from build123d import *

# Parameters (mm, degrees)
SKETCH1_W               = 406.4
SKETCH1_H               = 406.4
BOSS_EXTRUDE1_DEPTH     = 6.35
SKETCH2_R               = 50.8
CUT_EXTRUDE1_DEPTH      = 6.35
SKETCH3_W               = 406.4
SKETCH3_H               = 254
BOSS_EXTRUDE4_DEPTH     = 12.7
SKETCH6_R               = 50.8
CUT_EXTRUDE3_DEPTH      = 288.998927949
SKETCH7_R               = 7.14375
CUT_EXTRUDE4_DEPTH      = 288.648691984
F_1_2_20_TAPPED_HOLE1_D = 11.50874
SKETCH11_R              = 7.14375
CUT_EXTRUDE5_DEPTH      = 288.998927949


with BuildPart() as part:
    # Sketch1 → Boss-Extrude1 (new body)
    with BuildSketch(Plane(origin=(0, 0, 0), x_dir=(1, 0, 0), z_dir=(0, 1, 0))):
        Rectangle(SKETCH1_W, SKETCH1_H)
    extrude(amount=BOSS_EXTRUDE1_DEPTH)

    # Sketch2 → Cut-Extrude1 (cut)
    with BuildSketch(Plane(origin=(0, 6.35, 0), x_dir=(1, 0, 0), z_dir=(0, 1, 0))):
        with Locations(Location((-50.8, -55.88, 0), (0, 0, 270))):
            Circle(SKETCH2_R)
    extrude(amount=-CUT_EXTRUDE1_DEPTH, mode=Mode.SUBTRACT)

    # Sketch3 → Boss-Extrude4 (add)
    with BuildSketch(Plane(origin=(0, 6.35, 0), x_dir=(1, 0, 0), z_dir=(0, 1, 0))):
        with Locations((0, 76.2)):
            Rectangle(SKETCH3_W, SKETCH3_H)
    extrude(amount=BOSS_EXTRUDE4_DEPTH)

    # Sketch6 → Cut-Extrude3 (cut, through all)
    with BuildSketch(Plane.XZ):
        with Locations(Location((-50.8, 55.88, 0), (0, 0, 90))):
            Circle(SKETCH6_R)
    extrude(amount=-CUT_EXTRUDE3_DEPTH, mode=Mode.SUBTRACT)

    # Sketch7 → Cut-Extrude4 (cut, through all)
    with BuildSketch(Plane(origin=(0, 6.35, 0), x_dir=(1, 0, 0), z_dir=(0, 1, 0))):
        with Locations(Location((174.625, -182.5625, 0), (0, 0, 270))):
            Circle(SKETCH7_R)
        with Locations(Location((127, -182.5625, 0), (0, 0, 270))):
            Circle(SKETCH7_R)
        with Locations(Location((-174.625, -182.5625, 0), (0, 0, 270))):
            Circle(SKETCH7_R)
        with Locations(Location((-127, -182.5625, 0), (0, 0, 270))):
            Circle(SKETCH7_R)
    extrude(amount=-CUT_EXTRUDE4_DEPTH, mode=Mode.SUBTRACT)

    # 1/2-20 Tapped Hole1 (through all)
    with Locations(Plane(origin=(0, 19.05, 0), x_dir=(1, 0, 0), z_dir=(0, 1, 0))):
        with Locations((-174.625, 182.5625), (-127, 182.5625)):
            Hole(F_1_2_20_TAPPED_HOLE1_D / 2)

    # Sketch11 → Cut-Extrude5 (cut, through all)
    with BuildSketch(Plane(origin=(0, 19.05, 0), x_dir=(1, 0, 0), z_dir=(0, 1, 0))):
        with Locations(Location((174.625, 182.5625, 0), (0, 0, 270))):
            Circle(SKETCH11_R)
        with Locations(Location((127, 182.5625, 0), (0, 0, 270))):
            Circle(SKETCH11_R)
    extrude(amount=-CUT_EXTRUDE5_DEPTH, mode=Mode.SUBTRACT)


solid = part.part
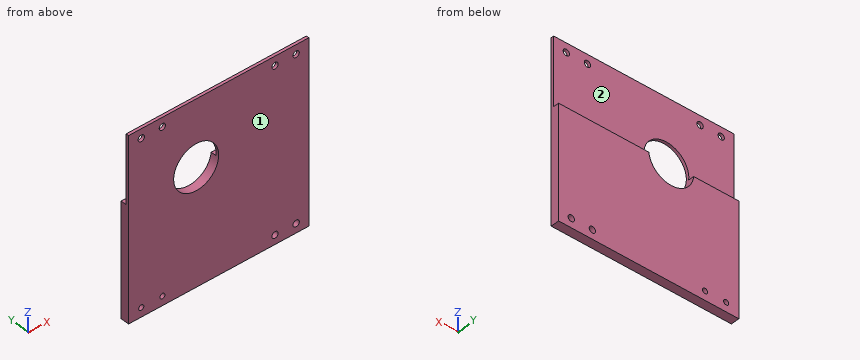
Read the model definition and answer for the solid it produces. Units are mm, in the model's axes. Face numbers are marked on the shaded views. A direction names the side the tool comes from. Give positions to 0.01 mm unless a question says otherwise; leave off trailing zeros. Write each loop counter-clockwise with the first axis right and the second up, starting at its lowest first coordinate (ties: lowest second). Pieces come first, ordered by that corner, then holes. Notation, with made-up numbers: (-11, 22.25) - (2, 22.25) arc R4 ccw to (2, 27.25) - close; hole circle Ø11 at (73.5, 58.25). An arc over 180 degrees is marked (long way). Answer in a Markdown table with one row per item. Add a question column.
Item 1: Section A-A, the plane x = 127 is taken. Write down the section's boundary in (y, z), and give its area (3 significant figures).
Item 2: Section C-C, the plane x = -50.8 is taken. Write down the section's boundary in (y, z), and give its area (3 significant figures).
Item 3: Section D-D, the plane y = 12.75 is taken. Write down the section's boundary in (x, z) (1 decimal), and give its area (3 significant figures).
Item 4: Section B-B, the plane z = 55.88 is taken. Write down the section's boundary in (x, y).
Item 5: Flat-ended cylindrical pins translate along their axes: P1, Ø11.5, axis at x = 127, z = 182.56, coming from the -Y side; P2, Ø16.5, axis at x = -174.62, z = 182.56, coming from the +Y side; P3, Ø6.5, axis at x = -129.5, y = 14, coming from the +Z side. Find the tip coordinate at first contact, or state that the pin passes through.
Item 6: Find the intervals of material crossed by L1, parallel to X at y = 1.75, z = 186; L2, parallel to Z at x = 131, y = 6.25; L3, parallel to Y at x = -27, z = 101, in increasing order.
Item 7: A tool of negligible diameter and unlimited length cuts with its end or side. For the marked faces 1 and 2, from which of +Z, -Z, +X, -X, +Y, -Y can it reach the whole face along a straight path? Write none if from no direction.
Recorded:
| question | item | result |
|---|---|---|
| 1 | outline | (0, -203.2) - (19.05, -203.2) - (19.05, -189.71) - (0, -189.71) - close; (0, -175.42) - (19.05, -175.42) - (19.05, 50.8) - (6.35, 50.8) - (6.35, 175.42) - (0, 175.42) - close; (0, 189.71) - (6.35, 189.71) - (6.35, 203.2) - (0, 203.2) - close |
| 1 | area | 5,440 mm2 |
| 2 | outline | (0, -203.2) - (19.05, -203.2) - (19.05, 5.08) - (0, 5.08) - close; (0, 106.68) - (6.35, 106.68) - (6.35, 203.2) - (0, 203.2) - close |
| 2 | area | 4,580 mm2 |
| 3 | outline | (-203.2, -203.2) - (203.2, -203.2) - (203.2, 50.8) - (-0.3, 50.8) arc R50.8 cw to (-101.3, 50.8) - (-203.2, 50.8) - close; hole circle Ø11.5 at (-174.6, -182.6); hole circle Ø11.5 at (-127, -182.6); hole circle Ø14.3 at (127, -182.6); hole circle Ø14.3 at (174.6, -182.6) |
| 3 | area | 99,200 mm2 |
| 4 | outline | (-203.2, 0) - (-101.6, 0) - (-101.6, 6.35) - (-203.2, 6.35) - close; (0, 0) - (203.2, 0) - (203.2, 6.35) - (0, 6.35) - close |
| 5 | P1 | passes through |
| 5 | P2 | stops at y = 6.35 |
| 5 | P3 | stops at z = 50.8 |
| 6 | L1 | x = -203.2 to -180.89, -168.36 to -133.26, -120.74 to 120.74, 133.26 to 168.36, 180.89 to 203.2 |
| 6 | L2 | z = -203.2 to -188.48, -176.64 to 176.64, 188.48 to 203.2 |
| 6 | L3 | y = 0 to 6.35 |
| 7 | face 1 | +Z, -Z, +X, -X, -Y |
| 7 | face 2 | +Z, +X, -X, +Y |
